Read the model definition and answer for the solid it produces. Units are mm, in the model's axes. Face numbers are marked on the shaded views. Give positions to 0.01 mm unless a question says otherwise; leave off trailing zeros. Write each loop counter-clockwise with the first axis right and the second up, starting at its lowest first coordinate (ties: lowest second). Pieces come first, ordered by that corner, then holes. Notation, with made-up numbers: (21, 88.25) -> (28, 88.25) arc R15 ccw to (28, 109.25) -> close; hole circle Ø1 at (23, 81). An arc over 180 degrees is marked (long way). Write item = value, one per line.
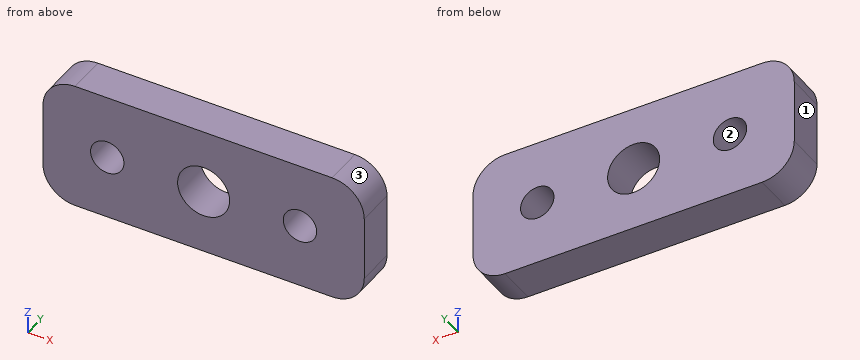
from build123d import *

# Parameters (mm, degrees)
ESBO_O1_W                = 50
ESBO_O1_H                = 20
RESSALTO_EXTRUS_O1_DEPTH = 3
ESBO_O3_R                = 4.05
ESBO_O3_R_2              = 2.6
CORTE_EXTRUS_O1_DEPTH    = 6
FILETE1_R                = 5


with BuildPart() as part:
    # Esboço1 → Ressalto-extrusão1 (new, symmetric)
    with BuildSketch(Plane(origin=(0, 0, 0), x_dir=(1, 0, 0), z_dir=(0, 1, 0))):
        Rectangle(ESBO_O1_W, ESBO_O1_H)
    extrude(amount=RESSALTO_EXTRUS_O1_DEPTH, both=True)

    # Esboço3 → Corte-extrusão1 (cut)
    with BuildSketch(Plane(origin=(0, 3, 0), x_dir=(1, 0, 0), z_dir=(0, 1, 0))):
        with Locations(Location((0, 0, 0), (0, 0, 270))):
            Circle(ESBO_O3_R)
        with Locations(Location((-15, 0, 0), (0, 0, 270))):
            Circle(ESBO_O3_R_2)
        with Locations(Location((15, 0, 0), (0, 0, 90))):
            Circle(ESBO_O3_R_2)
    extrude(amount=-CORTE_EXTRUS_O1_DEPTH, mode=Mode.SUBTRACT)

    # Filete1
    filete1_edges = [part.edges().sort_by_distance(p)[0] for p in [
        (25, 0, 10),
        (-25, 0, 10),
        (-25, 0, -10),
        (25, 0, -10),
    ]]
    fillet(filete1_edges, radius=FILETE1_R)


solid = part.part
(1) The part is cut by section D-D on x = 15. Determine the outline of the cut face in (y, z), plus the area to 3 significant figures.
Checks:
outline = (-3, -10) -> (3, -10) -> (3, -2.6) -> (-3, -2.6) -> close; (-3, 2.6) -> (3, 2.6) -> (3, 10) -> (-3, 10) -> close
area = 88.8 mm²
(2) The part is cut by section A-A on x = 0. Determine the outline of the cut face in (y, z).
Checks:
outline = (-3, -10) -> (3, -10) -> (3, -4.05) -> (-3, -4.05) -> close; (-3, 4.05) -> (3, 4.05) -> (3, 10) -> (-3, 10) -> close
(3) The part is cut by section C-C on y = 2.5. Determine the outline of the cut face in (x, z).
Checks:
outline = (-25, -5) arc R5 ccw to (-20, -10) -> (20, -10) arc R5 ccw to (25, -5) -> (25, 5) arc R5 ccw to (20, 10) -> (-20, 10) arc R5 ccw to (-25, 5) -> close; hole circle Ø5.2 at (-15, 0); hole circle Ø8.1 at (0, 0); hole circle Ø5.2 at (15, 0)
(4) The part is cut by section B-B on z = 0. Determine the outline of the cut face in (x, y), plus the area to 3 significant figures.
Checks:
outline = (-25, -3) -> (-17.6, -3) -> (-17.6, 3) -> (-25, 3) -> close; (-12.4, -3) -> (-4.05, -3) -> (-4.05, 3) -> (-12.4, 3) -> close; (4.05, -3) -> (12.4, -3) -> (12.4, 3) -> (4.05, 3) -> close; (17.6, -3) -> (25, -3) -> (25, 3) -> (17.6, 3) -> close
area = 189 mm²
(5) For a pull along Z with two mould halves and no side action, classify the marked faces 1, 2 and 3 as released by +Z, released by -Z, zero draft, split by the parting line, or undercut.
Checks:
face_1 = zero draft
face_2 = undercut
face_3 = released by +Z
(6) Consider L1, parallel to X at y = -1.3, z = 0; L2, parallel to Z at x = 15, y = 1.1; L3, parallel to Z at x = -13.5, y = -1.9. Determine where each line is inside the solid, lowest interval first.
Checks:
L1 = -25 to -17.6, -12.4 to -4.05, 4.05 to 12.4, 17.6 to 25
L2 = -10 to -2.6, 2.6 to 10
L3 = -10 to -2.12, 2.12 to 10
(7) Given P1, Ø4.5, axis at x = 15, z = 0, coming from the -Y side, flat-ended and moving along its own axis, determine where the tip first touches the part or whether it passes through.
Checks:
P1 = through
